Drawing for the job (mm, zero at the part's lowest x, y, z). A direction names the side the tool comes from. Give positions to 0.01 mm unless a question says otherwise; leave off trailing zeros. Loops run counter-clockwise (first coordinate to the right, second up) from the corner with the lowest first, then second, coordinate; pieces in that order, holes last.
1) Band-saw the part on B-B on x = 7.5. List the corners of the cut face in (y, z) (3 decimals), then the cut area to 3 significant figures.
2) Two-plate mould, pull along Y, no slides. Class the marked faces 6, 7, 8 and 9: +Y half, -Y half, draft (parallel to the pull), parting line (faces both ways), or undercut.
3) Band-saw the part on A-A on y = 27. List the corners of the cut face in (x, z) (3 decimals).
4) Band-saw the part on C-C on y = 19. List the corners of the cut face in (x, z) (3 decimals).
5) Wall check: line 1 (Z direction, x = 2.25, y = 18) (3 decimals); line 2 (X direction, y = 44.45, z = 11.9); line 3 (Y direction, x = 3.25, z = 9.25) (3 decimals). Give the ranges that are in metal, low to high.
6) 3-axis set-ups, long thin cutter, end or side, ignore diameter. For the marked faces 1, 2, 3, 4 and 5: which of +Z, -Z, +X, -X, +Y, -Y reach the whole face in a straight line?
7) Flat gauge pins, fed straight in: P1, Ø1.2, axis at x = 23, z = 8.5, coming from the +Y side; P2, Ø0.6, axis at y = 32, z = 3, coming from the +X side (3 decimals); P3, Ø1, axis at y = 31.5, z = 3, coming from the -X side (3 decimals); P4, Ø3.5, axis at x = 12.7, y = 6.35, coming from the -Z side. Where does each tip first touch, or does it go through?
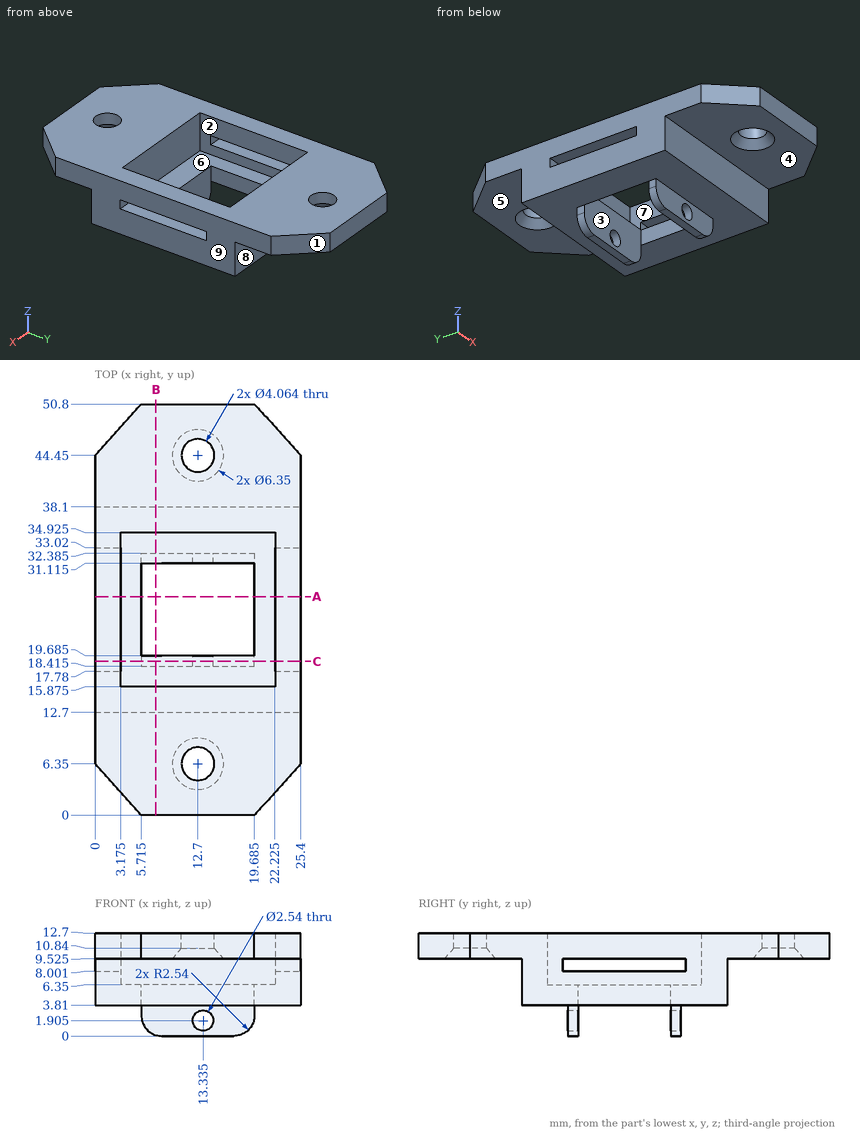
Findings below:
1. outline: (0, 9.525) - (12.7, 9.525) - (12.7, 3.81) - (18.415, 3.81) - (18.415, 0.115) - (19.685, 0.115) - (19.685, 6.35) - (15.875, 6.35) - (15.875, 12.7) - (0, 12.7) - close; (31.115, 0.115) - (32.385, 0.115) - (32.385, 3.81) - (38.1, 3.81) - (38.1, 9.525) - (50.8, 9.525) - (50.8, 12.7) - (34.925, 12.7) - (34.925, 6.35) - (31.115, 6.35) - close
1. area: 166 mm2
2. face 6: undercut
2. face 7: undercut
2. face 8: +Y half
2. face 9: draft
3. outline: (0, 3.81) - (5.715, 3.81) - (5.715, 6.35) - (3.175, 6.35) - (3.175, 8.001) - (0, 8.001) - close; (0, 9.525) - (3.175, 9.525) - (3.175, 12.7) - (0, 12.7) - close; (19.685, 3.81) - (25.4, 3.81) - (25.4, 8.001) - (22.225, 8.001) - (22.225, 6.35) - (19.685, 6.35) - close; (22.225, 9.525) - (25.4, 9.525) - (25.4, 12.7) - (22.225, 12.7) - close
4. outline: (0, 3.81) - (5.715, 3.81) - (5.715, 2.54) arc R2.54 ccw to (8.255, 0) - (17.145, 0) arc R2.54 ccw to (19.685, 2.54) - (19.685, 3.81) - (25.4, 3.81) - (25.4, 8.001) - (22.225, 8.001) - (22.225, 6.35) - (3.175, 6.35) - (3.175, 8.001) - (0, 8.001) - close; (0, 9.525) - (3.175, 9.525) - (3.175, 12.7) - (0, 12.7) - close; (22.225, 9.525) - (25.4, 9.525) - (25.4, 12.7) - (22.225, 12.7) - close; hole circle Ø2.54 at (13.335, 1.905)
5. line 1: z = 3.81 to 8.001, 9.525 to 12.7
5. line 2: x = 0 to 10.67, 14.73 to 25.4
5. line 3: y = 12.7 to 15.875, 34.925 to 38.1
6. face 1: +Z, -Z, +X, +Y
6. face 2: +Z
6. face 3: +Z, -Z
6. face 4: -Z, +X, -X, -Y
6. face 5: -Z, +X, -X, +Y
7. P1: stops at y = 38.1
7. P2: stops at x = 19.685
7. P3: stops at x = 5.715
7. P4: passes through
